from build123d import *

# Parameters (mm, degrees)
F0_R     = 18.4
F0_R_2   = 1.4
F0_R_3   = 11
F1_DEPTH = 4
F2_R     = 1.85
F3_DEPTH = 25
F5_DEPTH = 25


with BuildPart() as f1:
    # F0 (on Front) → F1 (new body)
    with BuildSketch(Plane.XZ):
        Circle(F0_R)
        with Locations((-8.25, -11.3551508439)):
            Circle(F0_R_2, mode=Mode.SUBTRACT)
        with Locations((8.25, -11.3551508439)):
            Circle(F0_R_2, mode=Mode.SUBTRACT)
        with Locations((-13.3487804072, 4.337281675)):
            Circle(F0_R_2, mode=Mode.SUBTRACT)
        Circle(F0_R_3, mode=Mode.SUBTRACT)
        with Locations((13.3487804072, 4.337281675)):
            Circle(F0_R_2, mode=Mode.SUBTRACT)
        with Locations((0, 14.0357383378)):
            Circle(F0_R_2, mode=Mode.SUBTRACT)
    extrude(amount=-F1_DEPTH)

    # F2 (on face) → F3 (cut)
    with BuildSketch(Plane(origin=(0, 4, 0), x_dir=(-1, 0, 0), z_dir=(0, 1, 0))):
        with Locations((0, -15.4548132206)):
            Circle(F2_R)
        with Locations((13.3842608598, -7.7274066103)):
            Circle(F2_R)
        with Locations((-13.3842608598, -7.7274066103)):
            Circle(F2_R)
        with Locations((-7.7274066103, 13.3842608598)):
            Circle(F2_R)
        with Locations((7.7274066103, 13.3842608598)):
            Circle(F2_R)
    extrude(amount=-F3_DEPTH, mode=Mode.SUBTRACT)

    # F4 (on face) → F5 (cut)
    with BuildSketch(Plane.XZ):
        with BuildLine():
            ThreePointArc((-18.2913043478, -1.9970441295), (-16.9478651398, -1.3752470134), (-16.4, 0))
            ThreePointArc((-16.4, 0), (-16.9478651398, 1.3752470134), (-18.2913043478, 1.9970441295))
            ThreePointArc((-18.2913043478, 1.9970441295), (-18.4, 0), (-18.2913043478, -1.9970441295))
        make_face()
        with BuildLine():
            ThreePointArc((18.4, 0), (18.3728059915, 1), (18.2913043478, 1.9970441295))
            ThreePointArc((18.2913043478, 1.9970441295), (16.4, 0), (18.2913043478, -1.9970441295))
            ThreePointArc((18.2913043478, -1.9970441295), (18.3728059915, -1), (18.4, 0))
        make_face()
    extrude(amount=-F5_DEPTH, mode=Mode.SUBTRACT)


solid = f1.part
Geometry: final body of the model. Coordinates: model frame, mm. Coordinates: 2 decimals unless noted, no trailing zeros. Loops run counter-clockwise (first coordinate to the right, second up) from the corner with the lowest first, then second, coordinate; pieces in that order, holes last. Notation, with made-up numbers: M 64.5,8 L 87.5,8 A5 cw 87.5,15 Z; hole C 59.25,-32 d8. An arc over 180 degrees is marked long. One line per item, written item: value. Start each with the question number.
1) Cut plane B-B (z = 1.5). Return loops of the section in (x, y), then the cut area to 3 significant figures.
2) Cut plane D-D (x = 5). Return loops of the section in (y, z), then the cut area to 3 significant figures.
3) Draft query along Z for faces 1 (the cylindrical face through (-0.377, 1.972, -18.396)), 2 (the cylindrical face through (0.377, 1.972, 18.396)), 3 (the flat face through (8, 0, 8)), 4 (the cylindrical face through (-14.747, 1.972, 4.399)). Return one class per face: released by +Z, released by -Z, zero draft, split by the parting line, or undercut.
4) Cut plane A-A (x = 0). Return loops of the section in (y, z), then the cut area to 3 significant figures.
5) Pin query (flat end, axial travel): P1, Ø10, axis at x = -6.5, z = -4, coming from the +Y side; P2, Ø1.5, axis at y = 1, z = 0, coming from the +X side. Return the tip coordinate at first contact, or that it passes through.
6) Material intervals for L1, parallel to Z at x = 0, y = 2.15; L2, parallel to Z at x = 8.25, y = 3; L3, parallel to X at y = 1.4, z = 5, sorted ascending. Write a range as from..to.
7) Cut plane C-C (z = 14.5). Return loops of the section in (x, y).
Evaluation:
1. outline: M -17.08,0 L -10.9,0 L -10.9,4 L -17.08,4 Z; M 10.9,0 L 17.08,0 L 17.08,4 L 10.9,4 Z
1. area: 49.4 mm^2
2. outline: M 0,-17.71 L 4,-17.71 L 4,-9.8 L 0,-9.8 Z; M 0,9.8 L 4,9.8 L 4,17.71 L 0,17.71 Z
2. area: 63.3 mm^2
3. face 1: released by -Z
3. face 2: released by +Z
3. face 3: zero draft
3. face 4: undercut
4. outline: M 0,-18.4 L 4,-18.4 L 4,-17.3 L 0,-17.3 Z; M 0,-13.6 L 4,-13.6 L 4,-11 L 0,-11 Z; M 0,11 L 4,11 L 4,12.64 L 0,12.64 Z; M 0,15.44 L 4,15.44 L 4,18.4 L 0,18.4 Z
4. area: 33.2 mm^2
5. P1: y = 4
5. P2: x = 16.55
6. L1: -18.4..-17.3, -13.6..-11, 11..12.64, 15.44..18.4
6. L2: -16.45..-12.76, -9.96..-7.28, 7.28..11.61, 15.16..16.45
6. L3: -17.71..-14.58, -12.12..-9.8, 9.8..12.12, 14.58..17.71
7. outline: M -11.33,0 L -9.2,0 L -9.2,4 L -11.33,4 Z; M -6.25,0 L -1.32,0 L -1.32,4 L -6.25,4 Z; M 1.32,0 L 6.25,0 L 6.25,4 L 1.32,4 Z; M 9.2,0 L 11.33,0 L 11.33,4 L 9.2,4 Z
